```python
from build123d import *

# Parameters (mm, degrees)
SKETCH1_R           = 1.6
BOSS_EXTRUDE1_DEPTH = 4.7625


with BuildPart() as part:
    # Sketch1 → Boss-Extrude1 (new body)
    with BuildSketch(Plane(origin=(0, 0, 0), x_dir=(1, 0, 0), z_dir=(0, 1, 0))):
        with BuildLine():
            Line((28.033109467, 7.5), (28.033109467, -7.5))
            Line((28.033109467, -7.5), (3.033109467, -7.5))
            ThreePointArc((3.033109467, -7.5), (-1.837792139, -6.858733638), (-6.376749851, -4.978635795))
            Line((-6.376749851, -4.978635795), (-28.027384945, 7.521364205))
            Line((-28.027384945, 7.521364205), (-20.527384945, 20.511745262))
            Line((-20.527384945, 20.511745262), (1.123250149, 8.011745262))
            ThreePointArc((1.123250149, 8.011745262), (2.044493537, 7.630153756), (3.033109467, 7.5))
            Line((3.033109467, 7.5), (28.033109467, 7.5))
        make_face()
        with Locations((23.033109467, 0)):
            Circle(SKETCH1_R, mode=Mode.SUBTRACT)
        with Locations((8.033109467, 0)):
            Circle(SKETCH1_R, mode=Mode.SUBTRACT)
        with Locations((-19.947257926, 11.516554733)):
            Circle(SKETCH1_R, mode=Mode.SUBTRACT)
        with Locations((-6.956876869, 4.016554733)):
            Circle(SKETCH1_R, mode=Mode.SUBTRACT)
    extrude(amount=BOSS_EXTRUDE1_DEPTH)


solid = part.part
```
Read the model definition and answer for the solid it produces. Units are mm, in the model's axes. A direction names the side the tool comes from. Coordinates: 2 decimals unless noted, no trailing zeros. Loops run counter-clockwise (first coordinate to the right, second up) from the corner with the lowest first, then second, coordinate; pieces in that order, holes last.
(1) Consider line 1 along X through (y, z) = (3.35, 0); line 2 along X through (y, z) = (2, 0.25); line 3 along Z through (x, y) = (15, 3.6). Determine where each line is inside the solid, lowest interval first.
Solution:
line 1: x = -15 to 6.43, 9.63 to 21.43, 24.63 to 28.03
line 2: x = -14.57 to 6.45, 9.61 to 21.45, 24.61 to 28.03
line 3: z = -7.5 to 7.5
(2) The part is cut by section C-C (y = 2.5). Determine the outline of the cut face in (x, z), and give its area (3 significant figures).
Solution:
outline: (-28.03, -7.52) - (-20.53, -20.51) - (1.12, -8.01) arc R3.82 cw to (3.03, -7.5) - (28.03, -7.5) - (28.03, 7.5) - (3.03, 7.5) arc R18.82 ccw to (-6.38, 4.98) - close; hole circle Ø3.2 at (-19.95, -11.52); hole circle Ø3.2 at (-6.96, -4.02); hole circle Ø3.2 at (8.03, 0); hole circle Ø3.2 at (23.03, 0)
area: 807 mm2
(3) A tool of negligible diameter and unlimited length cuts with its end or side. For faces 1 (the face through (15, 2, -7.5)), 2 (the face through (6.435, 2.348, -0.07)), from which of +Z, -Z, +X, -X, +Y, -Y can it reach the whole face along a straight path? Write none if from no direction.
Solution:
face 1: -Z, +X, +Y, -Y
face 2: +Y, -Y
(4) The part is cut by section A-A (z = 0). Determine the outline of the cut face in (x, y).
Solution:
outline: (-15, 0) - (6.43, 0) - (6.43, 4.76) - (-15, 4.76) - close; (9.63, 0) - (21.43, 0) - (21.43, 4.76) - (9.63, 4.76) - close; (24.63, 0) - (28.03, 0) - (28.03, 4.76) - (24.63, 4.76) - close
(5) The part is cut by section B-B (x = -7.5). Determine the outline of the cut face in (y, z), and give its area (3 significant figures).
Solution:
outline: (0, -12.99) - (4.76, -12.99) - (4.76, -5.52) - (0, -5.52) - close; (0, -2.51) - (4.76, -2.51) - (4.76, 4.33) - (0, 4.33) - close
area: 68.2 mm2
(6) The mould has two halves that part along Z. Classify faces 3 (the face through (-9.854, 2.348, -14.349)), 4 (the face through (-21.217, 2.348, -10.543)), 5 (the face through (28.033, 2, 0)), 6 (the face through (24.56, 2.35, -0.48)): released by +Z, released by -Z, zero draft, split by the parting line, or undercut.
Solution:
face 3: released by -Z
face 4: undercut
face 5: zero draft
face 6: undercut
(7) The part is cut by section D-D (x = 20). Determine the outline of the cut face in (y, z).
Solution:
outline: (0, -7.5) - (4.76, -7.5) - (4.76, 7.5) - (0, 7.5) - close
(8) Flat-ended cylindrical pins translate along their axes: pin 1 Ø4 at (x, z) = (-6.96, -4.02) entering from +Y; pin 2 Ø2.5 at (x, z) = (8.03, 0) entering from +Y; pin 3 Ø1 at (x, y) = (22, 0.5) entering from -Z. Find the tip coordinate at first contact, or state that the pin passes through.
Solution:
pin 1: stops at y = 4.76
pin 2: passes through
pin 3: stops at z = -7.5
